```python
from build123d import *

# Parameters (mm, degrees)
BOSS_EXTRUDE1_DEPTH = 90
FILLET1_R           = 1
FILLET2_R           = 2
SKETCH2_R           = 1.6
CUT_EXTRUDE1_DEPTH  = 10


with BuildPart() as part:
    # Sketch1 → Boss-Extrude1 (new body)
    with BuildSketch(Plane.XY):
        Polygon((1262.507506827, -206.048661528), (1262.507506827, -256.048661528), (1250.507506827, -256.048661528), (1250.507506827, -254.048661528), (1260.507506827, -254.048661528), (1260.507506827, -206.048661528), align=None)
    extrude(amount=BOSS_EXTRUDE1_DEPTH)

    # Fillet1
    fillet1_edges = [part.edges().sort_by_distance(p)[0] for p in [
        (1250.507506827, -254.048661528, 45),
        (1260.507506827, -206.048661528, 45),
    ]]
    fillet(fillet1_edges, radius=FILLET1_R)

    # Fillet2
    fillet2_edges = [part.edges().sort_by_distance(p)[0] for p in [
        (1260.507506827, -254.048661528, 45),
    ]]
    fillet(fillet2_edges, radius=FILLET2_R)

    # Sketch2 → Cut-Extrude1 (cut)
    with BuildSketch(Plane(origin=(0, -254.048661528, 0), x_dir=(1, 0, 0), z_dir=(0, 1, 0))):
        with Locations(Location((1255.007506827, -70, 0), (0, 0, 270))):
            Circle(SKETCH2_R)
        with Locations(Location((1255.007506827, -20, 0), (0, 0, 270))):
            Circle(SKETCH2_R)
    extrude(amount=-CUT_EXTRUDE1_DEPTH, mode=Mode.SUBTRACT)


solid = part.part
```
Verification items for the finished model (mm, model axes). A direction names the side the tool comes from. Coordinates: 2 decimals unless noted, no trailing zeros. Write each loop counter-clockwise with the first axis right and the second up, starting at its lowest first coordinate (ties: lowest second). Pieces come first, ordered by that corner, then holes. Notation, with made-up numbers: (-3, -25) - (41, -25) arc R29 cw to (41, 14) - close; hole circle Ø1 at (-24, 55.5). An arc over 180 degrees is marked (long way). One line per question, with ' | ' between items. Start each with the question number.
1. Section check B-B (y = -228.5). Enter the section's corners in (x, z).
2. Section check A-A (z = 70). Enter the section's corners in (x, y), plus the area to 3 significant figures.
3. Draft check along X on faces 1 (the cylindrical face through (1256.594, -255.035, 69.792)), 2 (the flat face through (1257, -256.049, 44)), 3 (the cylindrical face through (1259.906, -253.478, 45.63)). Enter one of: released by +X, released by -X, zero draft, split by the parting line, or undercut.
4. Access from +Z, -Z, +X, -X, +Y, -Y to the whole of each face (thin tool, end or side, straight path). Record for faces 4 (the flat face through (1261, -235, 0)), 5 (the flat face through (1260.508, -230, 44)).
5. Gauge pin test, flat ends, axial feed: P1, Ø3.5, axis at x = 1256.5, z = 40.5, coming from the +Y side; P2, Ø12, axis at y = -232.5, z = 37.5, coming from the -X side. Record the tip position at first contact, or that the pin passes through.
6. Material ranges on line 1 along X through (y, z) = (-255.3, 70); line 2 along Y through (x, z) = (1255, 63); line 3 along X through (y, z) = (-254.45, 20), recorded low to high.
Computed values:
1) outline: (1260.51, 0) - (1262.51, 0) - (1262.51, 90) - (1260.51, 90) - close
2) outline: (1250.51, -256.05) - (1253.41, -256.05) - (1253.41, -254.05) - (1251.51, -254.05) arc R1 ccw to (1250.51, -255.05) - close; (1256.61, -256.05) - (1262.51, -256.05) - (1262.51, -206.05) - (1261.51, -206.05) arc R1 ccw to (1260.51, -207.05) - (1260.51, -252.05) arc R2 cw to (1258.51, -254.05) - (1256.61, -254.05) - close | area: 114 mm²
3) face 1: undercut | face 2: zero draft | face 3: released by -X
4) face 4: -Z, +X, -X, +Y, -Y | face 5: +Z, -Z, -X, +Y
5) P1: y = -254.05 | P2: x = 1260.51
6) line 1: 1250.51 to 1253.41, 1256.61 to 1262.51 | line 2: -256.05 to -254.05 | line 3: 1250.71 to 1253.41, 1256.61 to 1262.51
